Here's how the part is built. I have some questions about the finished solid (model axes, mm). Face numbers are marked on the shaded views. A direction names the side the tool comes from. Give positions to 0.01 mm unless a question says otherwise; leave off trailing zeros. Loops run counter-clockwise (first coordinate to the right, second up) from the corner with the lowest first, then second, coordinate; pieces in that order, holes last. Notation, with made-up numbers: (28.25, 53) - (43.25, 53) arc R19 ccw to (43.25, 87) - close; hole circle Ø5 at (86, -28). An arc over 180 degrees is marked (long way). Use one line per item in the form item = value.
from build123d import *
from build123d.topology import SkipClean

# Parameters (mm, degrees)
CUT_EXTRUDE1_DEPTH       = 10
CUT_EXTRUDE1_DEPTH_BACK  = 10
SKETCH2_R                = 1.5
BOSS_EXTRUDE1_DEPTH      = 2
BOSS_EXTRUDE1_DEPTH_BACK = 2
SKETCH4_W                = 33
SKETCH4_H                = 9
CUT_EXTRUDE2_DEPTH       = 1.5
CUT_EXTRUDE2_DEPTH_BACK  = 10
SKETCH5_R                = 1.5
CUT_EXTRUDE3_DEPTH       = 10
CUT_EXTRUDE3_DEPTH_BACK  = 10
SKETCH8_R                = 1.5
SKETCH9_W                = 8.987494889
SKETCH9_H                = 0.781338227
SKETCH9_H_2              = 1.225544695
CUT_EXTRUDE4_DEPTH       = 46
SKETCH10_W               = 5.5
SKETCH10_H               = 2
CUT_EXTRUDE5_DEPTH       = 30
SKETCH11_W               = 3
SKETCH11_H               = 9
BOSS_EXTRUDE2_DEPTH      = 7
SKETCH12_R               = 1.5
CUT_EXTRUDE6_DEPTH       = 7
FILLET1_R                = 1
FILLET2_R                = 1
FILLET3_R                = 1
FILLET4_R                = 1
SKETCH13_W               = 28.065917506
SKETCH13_H               = 13.293965236
CUT_EXTRUDE7_DEPTH       = 10


with BuildPart() as part:
    # Sketch1 → Revolve1 (revolve)
    with BuildSketch(Plane.XY):
        with BuildLine():
            Line((0, 0), (-6, 0))
            ThreePointArc((-6, 0), (-3, 3), (0, 0))
        make_face()
    revolve(axis=Axis((0, 0, 0), (-1, 0, 0)))

    # Sketch2 → Cut-Extrude1 (cut, two sides: drawn at the far end of the back side and taken through both)
    with BuildSketch(Plane(origin=(0, 0, 0), x_dir=(1, 0, 0), z_dir=(0, 1, 0)).offset(-CUT_EXTRUDE1_DEPTH_BACK)):
        with Locations(Location((-3, 0, 0), (0, 0, 90))):
            Circle(SKETCH2_R)
    extrude(amount=CUT_EXTRUDE1_DEPTH + CUT_EXTRUDE1_DEPTH_BACK, mode=Mode.SUBTRACT)

    # Sketch4 → Boss-Extrude1 (add, two sides: drawn at the far end of the back side and taken through both)
    with SkipClean():  # the faces are left unmerged after this step: merging them gives an invalid solid
        with BuildSketch(Plane(origin=(0, 0, 0), x_dir=(1, 0, 0), z_dir=(0, 1, 0)).offset(-BOSS_EXTRUDE1_DEPTH_BACK)):
            with Locations((-14, 0)):
                Rectangle(SKETCH4_W, SKETCH4_H)
        extrude(amount=BOSS_EXTRUDE1_DEPTH + BOSS_EXTRUDE1_DEPTH_BACK)

    # Sketch5 → Cut-Extrude2 (cut, two sides: drawn at the far end of the back side and taken through both)
    with SkipClean():  # the faces are left unmerged after this step: merging them gives an invalid solid
        with BuildSketch(Plane(origin=(0, 2, 0), x_dir=(1, 0, 0), z_dir=(0, 1, 0)).offset(-CUT_EXTRUDE2_DEPTH_BACK)):
            with Locations(Location((-3, 0, 0), (0, 0, 90))):
                Circle(SKETCH5_R)
        extrude(amount=CUT_EXTRUDE2_DEPTH + CUT_EXTRUDE2_DEPTH_BACK, mode=Mode.SUBTRACT)

    # Sketch6 → Cut-Revolve1 (revolve, cut)
    with BuildSketch(Plane(origin=(0, 0, 0), x_dir=(1, 0, 0), z_dir=(0, 1, 0))):
        with BuildLine():
            Line((-3, 3.5), (-3, -3.5))
            ThreePointArc((-3, -3.5), (-6.5, 0), (-3, 3.5))
        make_face()
    revolve(axis=Axis((-3, 0, -3.5), (0, 0, 1)), mode=Mode.SUBTRACT)

    # Sketch10 → Cut-Extrude5 (cut)
    with BuildSketch(Plane.ZY.offset(30.5)):
        Rectangle(SKETCH10_W, SKETCH10_H)
    extrude(amount=-CUT_EXTRUDE5_DEPTH, mode=Mode.SUBTRACT)

    # Sketch11 → Boss-Extrude2 (add)
    with BuildSketch(Plane(origin=(0, 2, 0), x_dir=(1, 0, 0), z_dir=(0, 1, 0))):
        with Locations((-29, 0)):
            Rectangle(SKETCH11_W, SKETCH11_H)
    extrude(amount=BOSS_EXTRUDE2_DEPTH)

    # Sketch12 → Cut-Extrude6 (cut)
    with BuildSketch(Plane(origin=(-27.5, 0, 0), x_dir=(0, 0, -1), z_dir=(1, 0, 0))):
        with Locations((0, 5.5)):
            Circle(SKETCH12_R)
    extrude(amount=-CUT_EXTRUDE6_DEPTH, mode=Mode.SUBTRACT)

    # Fillet1
    fillet1_edges = [part.edges().sort_by_distance(p)[0] for p in [
        (2.5, 0, -4.5),
    ]]
    fillet(fillet1_edges, radius=FILLET1_R)

    # Fillet2
    fillet2_edges = [part.edges().sort_by_distance(p)[0] for p in [
        (2.5, 0, 4.5),
    ]]
    fillet(fillet2_edges, radius=FILLET2_R)

    # Fillet3
    fillet3_edges = [part.edges().sort_by_distance(p)[0] for p in [
        (-27.5, 2, 0),
    ]]
    fillet(fillet3_edges, radius=FILLET3_R)

    # Fillet4
    fillet4_edges = [part.edges().sort_by_distance(p)[0] for p in [
        (-12.5, 2, 4.5),
        (-27.207106781, 2.292893219, -4.5),
        (-27.207106781, 2.292893219, 4.5),
        (-27.5, 6, 4.5),
        (-27.5, 6, -4.5),
        (-12.5, 2, -4.5),
        (2.207106781, 2, -4.207106781),
        (2.5, 2, 0),
        (2.207106781, 2, 4.207106781),
    ]]
    fillet(fillet4_edges, radius=FILLET4_R)


with BuildPart() as body_2:
    # Sketch7 → Revolve2 (revolve)
    with BuildSketch(Plane(origin=(0, 0, 0), x_dir=(1, 0, 0), z_dir=(0, 1, 0))):
        with BuildLine():
            Line((-3, 3), (-3, -3))
            ThreePointArc((-3, -3), (-6, 0), (-3, 3))
        make_face()
    revolve(axis=Axis((-3, 0, -3), (0, 0, 1)))

    # Sketch8 → Cut-Extrude3 (cut, two sides: drawn at the far end of the back side and taken through both)
    with BuildSketch(Plane(origin=(0, 0, 0), x_dir=(1, 0, 0), z_dir=(0, 1, 0)).offset(-CUT_EXTRUDE3_DEPTH_BACK)):
        with Locations(Location((-3, 0, 0), (0, 0, 90))):
            Circle(SKETCH8_R)
    extrude(amount=CUT_EXTRUDE3_DEPTH + CUT_EXTRUDE3_DEPTH_BACK, mode=Mode.SUBTRACT)

    # Sketch9 → Cut-Extrude4 (cut)
    with BuildSketch(Plane.ZY.offset(30.5)):
        with Locations((-0.006252555, 2.390669113)):
            Rectangle(SKETCH9_W, SKETCH9_H)
        with Locations((-0.006252555, -2.612772347)):
            Rectangle(SKETCH9_W, SKETCH9_H_2)
    extrude(amount=-CUT_EXTRUDE4_DEPTH, mode=Mode.SUBTRACT)


with BuildPart() as cut_extrude7_tool:
    # Sketch13 → Cut-Extrude7 (new body)
    with BuildSketch(Plane(origin=(0, 2, 0), x_dir=(1, 0, 0), z_dir=(0, 1, 0))):
        with Locations((-9.778349348, -0.92291484)):
            Rectangle(SKETCH13_W, SKETCH13_H)
    extrude(amount=-CUT_EXTRUDE7_DEPTH)


with BuildPart() as part_1:
    add(part.part)

    # Cut-Extrude7: cut by cut_extrude7_tool
    add(cut_extrude7_tool.part, mode=Mode.SUBTRACT)


with BuildPart() as body_2_1:
    add(body_2.part)

    # Cut-Extrude7: cut by cut_extrude7_tool
    add(cut_extrude7_tool.part, mode=Mode.SUBTRACT)


solid = part_1.part
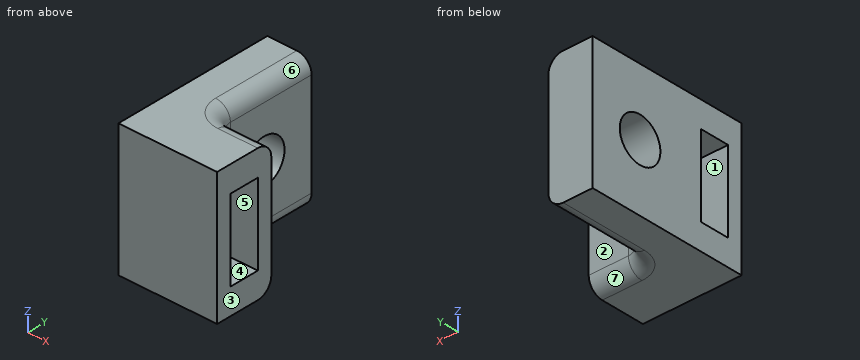
(1) If we section it at A-A (z = 0): List the corners of the cut face in (x, y) for me, plus the area to 3 significant figures.
Geometry says:
outline = (-30.5, -2) - (-23.81, -2) - (-23.81, -1) - (-30.5, -1) - close; (-30.5, 1) - (-23.81, 1) - (-23.81, 2) - (-26.5, 2) arc R1 cw to (-27.5, 3) - (-27.5, 4) - (-30.5, 4) - close; (-30.5, 7) - (-27.5, 7) - (-27.5, 9) - (-30.5, 9) - close
area = 25.6 mm²
(2) If we section it at C-C (z = -2.25): List the corners of the cut face in (x, y) for me.
Geometry says:
outline = (-30.5, -2) - (-23.81, -2) - (-23.81, -1) - (-30.5, -1) - close; (-30.5, 1) - (-23.81, 1) - (-23.81, 2) - (-26.5, 2) arc R1 cw to (-27.5, 3) - (-27.5, 9) - (-30.5, 9) - close
(3) For P1, Ø5, axis at y = 0.5, z = 0.5, coming from the -X side; P2, Ø2, axis at x = -25, z = 2, coming from the +Y side; P3, Ø4, axis at y = 6, z = 2.5, coming from the +X side, each with a flat end and sliding along its axis, tell me the tip position at first contact or that it passes through.
Geometry says:
P1 = -30.5
P2 = 2
P3 = -27.5
(4) If I drill on probe 1 along Y at (x, z) = (-28.7, 0); probe 2 along Y at (x, z) = (-26, -0.75); probe 3 along Y at (x, z) = (-29.5, 2), over which ranges is the centre line in solid material (lowest first)?
Geometry says:
probe_1 = -2 to -1, 1 to 4, 7 to 9
probe_2 = -2 to -1, 1 to 2
probe_3 = -2 to -1, 1 to 9
(5) If we section it at B-B (x = -24.75): List the corners of the cut face in (y, z) for me, plus the area to 3 significant figures.
Geometry says:
outline = (-2, -4.5) - (1, -4.5) arc R1 ccw to (2, -3.5) - (2, 3.5) arc R1 ccw to (1, 4.5) - (-2, 4.5) - close; hole (-1, -2.75) - (1, -2.75) - (1, 2.75) - (-1, 2.75) - close
area = 24.6 mm²
(6) For the marked faces 1, 2 and 3, which set-ups out of +Z, -Z, +X, -X, +Y, -Y let a thin tool reach every point of the face, with its end or its side?
Geometry says:
face_1 = +X, -X
face_2 = +Z, -Z, +X, +Y
face_3 = +Z, -Z, +X, +Y, -Y
(7) Thinking about a two-plate mould opening in Y: for the marked faces 4, 5, 6 and 7, which applies, pulls with the +Y half, pulls with the -Y half, needs draft (parallel to the pull), parting line crosses it, or undercut?
Geometry says:
face_4 = undercut
face_5 = undercut
face_6 = needs draft
face_7 = pulls with the +Y half
(8) If we section it at D-D (y = 5.5): List the corners of the cut face in (x, z) for me.
Geometry says:
outline = (-30.5, -4.5) - (-28.5, -4.5) arc R1 ccw to (-27.5, -3.5) - (-27.5, -1.5) - (-30.5, -1.5) - close; (-30.5, 1.5) - (-27.5, 1.5) - (-27.5, 3.5) arc R1 ccw to (-28.5, 4.5) - (-30.5, 4.5) - close
